from build123d import *

# Parameters (mm, degrees)
SKETCH1_R           = 50.8
SKETCH1_R_2         = 6.35
BOSS_EXTRUDE1_DEPTH = 15.875
SKETCH2_R           = 40.64
SKETCH2_R_2         = 12.7
CUT_EXTRUDE1_DEPTH  = 10.16
CUT_EXTRUDE2_REACH  = 77.016
SKETCH3_R           = 8.758928998


with BuildPart() as part:
    # Sketch1 → Boss-Extrude1 (new, symmetric)
    with BuildSketch(Plane.XY):
        Circle(SKETCH1_R)
        Circle(SKETCH1_R_2, mode=Mode.SUBTRACT)
    extrude(amount=BOSS_EXTRUDE1_DEPTH, both=True)

    # Sketch2 → Cut-Extrude1 (cut)
    with BuildSketch(Plane.XY.offset(15.875)):
        Circle(SKETCH2_R)
        Circle(SKETCH2_R_2, mode=Mode.SUBTRACT)
    cut_extrude1 = extrude(amount=-CUT_EXTRUDE1_DEPTH, mode=Mode.SUBTRACT)

    # Mirror1: Cut-Extrude1 across plane
    add(cut_extrude1.mirror(Plane.XY), mode=Mode.SUBTRACT)

    # Sketch3 → Cut-Extrude2 (cut, up to next)
    with BuildSketch(Plane.XY.offset(5.715), mode=Mode.PRIVATE) as cut_extrude2_sk1:
        with Locations((-23.151287749, -15.527256866)):
            Circle(SKETCH3_R)
    cut_extrude2_tool1 = extrude(cut_extrude2_sk1.sketch, amount=-CUT_EXTRUDE2_REACH, mode=Mode.PRIVATE) & part.part
    add(cut_extrude2_tool1.solids().sort_by_distance((-23.151288, -15.527257, 5.715))[0], mode=Mode.SUBTRACT)


solid = part.part
Could you check a few things on this model? Use its own coordinates, in mm. A direction names the side the tool comes from. Coordinates: 2 decimals unless noted, no trailing zeros. Loops run counter-clockwise (first coordinate to the right, second up) from the corner with the lowest first, then second, coordinate; pieces in that order, holes last.
1. We'd pull the mould along X, two halves only. Please class faces 1 (the face through (-11.012, -49.592, 0.222)), 2 (the face through (3, 6, 15.875)), 3 (the face through (-30.1, -20.86, 0.08)): released by +X, released by -X, zero draft, split by the parting line, or undercut.
2. For P1, Ø2, axis at x = 11, y = 36, coming from the +Z side (3 decimals); P2, Ø1, axis at x = -31.5, z = -12, coming from the -Y side; P3, Ø1.5, axis at x = 31, z = 2.5, coming from the -Y side, each with a flat end and sliding along its axis, tell me the tip position at first contact or that it passes through.
3. Imagine slicing it at D-D (x = -36.5). Please give me the cut outline in (y, z) (3 decimals).
4. Imagine slicing it at C-C (z = 7). Please give me the cut outline in (x, y), and give its area (3 significant figures).
5. Imagine slicing it at A-A (x = 0). Please give me the cut outline in (y, z) (3 decimals), and give its area (3 significant figures).
6. For faces 4 (the face through (-10, 10, -5.715)), 5 (the face through (-2.75, -12.4, 10.87)), 6 (the face through (-23, 34, -15.875)), which set-ups out of +Z, -Z, +X, -X, +Y, -Y let a thin tool reach every point of the face, with its end or its side?
7. I need wall thicknesses on L1, parallel to Y at x = 0, z = -8; L2, parallel to Y at x = 0, z = 1; L3, parallel to X at y = 9.5, z = -10.5. Which ranges of each line are inside material? Lowest first, please.
Computed values:
1. face 1: split by the parting line
1. face 2: zero draft
1. face 3: undercut
2. P1: stops at z = 5.715
2. P2: stops at y = -40.24
2. P3: stops at y = -40.81
3. outline: (-35.333, -15.875) - (-17.871, -15.875) - (-17.871, -5.715) - (17.871, -5.715) - (17.871, -15.875) - (35.333, -15.875) - (35.333, 15.875) - (17.871, 15.875) - (17.871, 5.715) - (-17.871, 5.715) - (-17.871, 15.875) - (-35.333, 15.875) - close
4. outline: circle Ø101.6 at (0, 0); circle Ø25.4 at (0, 0); hole circle Ø81.28 at (0, 0); hole circle Ø12.7 at (0, 0)
4. area: 3,300 mm2
5. outline: (-50.8, -15.875) - (-40.64, -15.875) - (-40.64, -5.715) - (-12.7, -5.715) - (-12.7, -15.875) - (-6.35, -15.875) - (-6.35, 15.875) - (-12.7, 15.875) - (-12.7, 5.715) - (-40.64, 5.715) - (-40.64, 15.875) - (-50.8, 15.875) - close; (6.35, -15.875) - (12.7, -15.875) - (12.7, -5.715) - (40.64, -5.715) - (40.64, -15.875) - (50.8, -15.875) - (50.8, 15.875) - (40.64, 15.875) - (40.64, 5.715) - (12.7, 5.715) - (12.7, 15.875) - (6.35, 15.875) - close
5. area: 1,690 mm2
6. face 4: -Z
6. face 5: +Z
6. face 6: -Z, +X, -X, +Y, -Y
7. L1: y = -50.8 to -40.64, -12.7 to -6.35, 6.35 to 12.7, 40.64 to 50.8
7. L2: y = -50.8 to -6.35, 6.35 to 50.8
7. L3: x = -49.9 to -39.51, -8.43 to 8.43, 39.51 to 49.9
